Geometry: see drawing. Coordinates: mm, zero at the bounding-box minimum. A direction names the side the tool comes from. Give positions to 0.01 mm unless a question says otherwise; leave off trailing zeros. Loops run counter-clockwise (first coordinate to the right, second up) from the corner with the lowest first, then second, coordinate; pieces in that order, holes last. Notation, with made-up numbers: (45.25, 56) -> (91.25, 56) arc R18 ccw to (91.25, 76) -> close; hole circle Ø1 at (28.25, -1.5). An arc over 180 degrees is marked (long way). Return JSON: item names as keys, results as strings. Group by question number.
(1) Draft query along Y for the marked faces 6, 7 and 8. Return one class per face: released by +Y, released by -Y, zero draft, split by the parting line, or undercut.
(2) Cut plane B-B on z = 93. Return loops of the section in (x, y), then the cut area to 3 significant figures.
(3) Access query for the marked faces 1, 2, 3, 4 and 5. Directions: +Z, -Z, +X, -X, +Y, -Y. A direction counts if a zero-diameter tool reaches every point of the face in a straight line with its end or side. Return the directions, or none.
(4) Cut plane C-C on x = 105. Return loops of the section in (y, z), then the cut area to 4 significant figures.
(5) Pin query (flat end, axial travel): pin 1 (14 mm diameter, centred on y = 86.5, z = 16.5, fed in from -X); pin 2 (12.5 mm diameter, centred on x = 71, z = 55, fed in from -Y); pin 3 (8 mm diameter, centred on y = 102, z = 52.5, fed in from +X) (3 decimals); pin 4 (2 mm diameter, centred on x = 144.5, y = 19, fed in from -Z). Return the tip coordinate at first contact, or that it passes through.
(6) Cut plane D-D on y = 99.5. Return loops of the section in (x, z).
(7) Cut plane A-A on y = 10. Return loops of the section in (x, z), then the cut area to 3 significant figures.
(8) Ray query, line 1 (X direction, y = 95.5, z = 19.5); line 2 (X direction, y = 132, z = 100.5); line 3 (Y direction, x = 144, z = 52). Return the intervals inside material, ascending. Write a range as from..to.
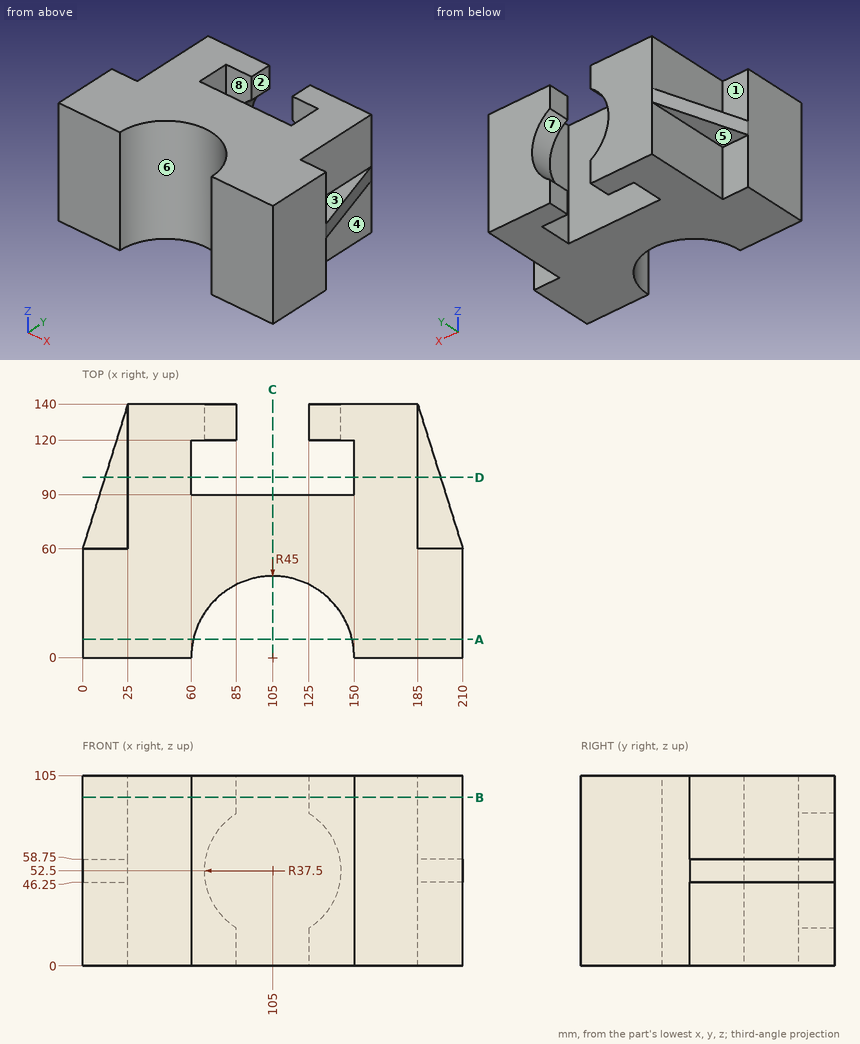
Answers:
{
 "1": {"face 6": "released by -Y", "face 7": "zero draft", "face 8": "undercut"},
 "2": {"outline": "(0, 0) -> (60, 0) arc R45 cw to (150, 0) -> (210, 0) -> (210, 60) -> (185, 60) -> (185, 140) -> (125, 140) -> (125, 120) -> (150, 120) -> (150, 90) -> (60, 90) -> (60, 120) -> (85, 120) -> (85, 140) -> (25, 140) -> (25, 60) -> (0, 60) -> close", "area": "18,700 mm²"},
 "3": {"face 1": "+Z, -X, +Y", "face 2": "+Z, -Z, +Y", "face 3": "+Z, +X, +Y", "face 4": "-Z, +X, +Y", "face 5": "-Z, -X, +Y"},
 "4": {"outline": "(45, 0) -> (90, 0) -> (90, 105) -> (45, 105) -> close", "area": "4,725 mm²"},
 "5": {"pin 1": "x = 25", "pin 2": "y = 20.12", "pin 3": "x = 198.125", "pin 4": "through"},
 "6": {"outline": "(12.34, 46.25) -> (25, 46.25) -> (25, 0) -> (60, 0) -> (60, 105) -> (25, 105) -> (25, 58.75) -> (12.34, 58.75) -> close; (150, 0) -> (185, 0) -> (185, 46.25) -> (197.66, 46.25) -> (197.66, 58.75) -> (185, 58.75) -> (185, 105) -> (150, 105) -> close"},
 "7": {"outline": "(0, 0) -> (61.13, 0) -> (61.13, 105) -> (0, 105) -> close; (148.87, 0) -> (210, 0) -> (210, 105) -> (148.87, 105) -> close", "area": "12,800 mm²"},
 "8": {"line 1": "25..60, 150..185", "line 2": "25..85, 125..185", "line 3": "22.45..90, 120..140"}
}
